from build123d import *

# Parameters (mm, degrees)
SKETCH_1_R          = 6
EXTRUDE_1_DEPTH     = 3
SKETCH_2_W          = 8
SKETCH_2_H          = 8
EXTRUDE_2_DEPTH     = 5.1
SKETCH_4_R          = 2.85
CUT_EXTRUDE_1_DEPTH = 1
SKETCH_5_R          = 1.55
CUT_EXTRUDE_2_DEPTH = 8.1


with BuildPart() as part:
    # 草图1 → 凸台-拉伸1 (new body)
    with BuildSketch(Plane.XY):
        Circle(SKETCH_1_R)
    extrude(amount=EXTRUDE_1_DEPTH)

    # 草图2 → 凸台-拉伸2 (add)
    with BuildSketch(Plane.XY.offset(3)):
        Rectangle(SKETCH_2_W, SKETCH_2_H)
    extrude(amount=EXTRUDE_2_DEPTH)

    # 草图4 → 切除-拉伸1 (cut)
    with BuildSketch(Plane(origin=(0, 0, 0), x_dir=(-1, 0, 0), z_dir=(0, 0, -1))):
        Circle(SKETCH_4_R)
    extrude(amount=-CUT_EXTRUDE_1_DEPTH, mode=Mode.SUBTRACT)

    # 草图5 → 切除-拉伸2 (cut, through all)
    with BuildSketch(Plane(origin=(0, 0, 1), x_dir=(-1, 0, 0), z_dir=(0, 0, -1))):
        Circle(SKETCH_5_R)
    extrude(amount=-CUT_EXTRUDE_2_DEPTH, mode=Mode.SUBTRACT)


solid = part.part
Design review of the part built by this model. Coordinates are the model's own, in mm. A direction names the side the tool comes from. Give positions to 0.01 mm unless a question says otherwise; leave off trailing zeros. Loops run counter-clockwise (first coordinate to the right, second up) from the corner with the lowest first, then second, coordinate; pieces in that order, holes last. Notation, with made-up numbers: M -14.5,-15 L 20.5,-15 A22 cw 20.5,3 Z; hole C -4,58 d9. An arc over 180 degrees is marked long. Write item = value, one per line.
Q1. Draft analysis for pull direction X (two halves, no side actions). For faces 1 (the cylindrical face through (2.262, -1.734, 0.493)), 2 (the flat face through (-2, 0, 8.1)), 3 (the flat face through (4, 0, 6)), state which applies: +X half, -X half, draft (parallel to the pull), parting line (faces both ways), or undercut.
Output values:
face_1 = undercut
face_2 = draft
face_3 = +X half
Q2. Insertion check: pin 1 (3 mm diameter, centred on y = 3, z = 1, fed in from +X); pin 2 (4 mm diameter, centred on x = -1.5, z = 4.5, fed in from +Y); pin 3 (4 mm diameter, centred on y = 0.5, z = 6, fed in from -X). Each pin has a flat end and moves straight along its axis. Give the tip position at first contact, or say it passes through.
Output values:
pin_1 = 5.81
pin_2 = 6
pin_3 = -4
Q3. We need section B-B (z = 3.75). Give the boundary of the cut face in (x, y).
Output values:
outline = M -4,-4 L 4,-4 L 4,4 L -4,4 Z; hole C 0,0 d3.1
Q4. We need section D-D (y = 3.5). Give the boundary of the cut face in (x, z), plus the area to 3 significant figures.
Output values:
outline = M -4.87,0 L 4.87,0 L 4.87,3 L 4,3 L 4,8.1 L -4,8.1 L -4,3 L -4.87,3 Z
area = 70.0 mm^2
Q5. For faces 4 (the flat face through (-4, 0, 6)), 5 (the flat face through (0, 4, 6)), 6 (the flat face through (-1.23, -1.23, 1)), 7 (the flat face through (0, -4, 6)), list the 3-axis set-ups (+Z, -Z, +X, -X, +Y, -Y) from which the entire face can be reached by the end or side of a thin tool; tool diameter is ignored.
Output values:
face_4 = +Z, -X, +Y, -Y
face_5 = +Z, +X, -X, +Y
face_6 = -Z
face_7 = +Z, +X, -X, -Y
Q6. We need section A-A (x = 0). Give the boundary of the cut face in (y, z).
Output values:
outline = M -6,0 L -2.85,0 L -2.85,1 L -1.55,1 L -1.55,8.1 L -4,8.1 L -4,3 L -6,3 Z; M 1.55,1 L 2.85,1 L 2.85,0 L 6,0 L 6,3 L 4,3 L 4,8.1 L 1.55,8.1 Z
Q7. To check wall thickness, follow line 1 (Y direction, x = 0, z = 0.2); line 2 (Y direction, x = 0, z = 5.25); line 3 (Y direction, x = 2.25, z = 6). State the ranges of each line that lie inside material, in increasing order. Write a range as [from, to].
Output values:
line_1 = [-6, -2.85], [2.85, 6]
line_2 = [-4, -1.55], [1.55, 4]
line_3 = [-4, 4]
